Autodesk Inventor part; units mm, degrees
ref_plane "YZ Plane" through (0, 0, 0) normal (1, 0, 0) x (0, 1, 0)
ref_plane "XZ Plane" through (0, 0, 0) normal (0, 1, 0) x (-1, 0, 0)
ref_plane "XY Plane" through (0, 0, 0) normal (0, 0, 1) x (1, 0, 0)
sketch "スケッチ1" plane through (0, 0, 0) normal (0, 0, 1) x (1, 0, 0)
  line L0 (-22.5, 3.5) -> (22.5, 3.5)
  line L1 (22.5, 3.5) -> (22.5, -3.5)
  line L2 (22.5, -3.5) -> (-22.5, -3.5)
  line L3 (-22.5, -3.5) -> (-22.5, 3.5)
  line L4 (-22.5, 3.5) -> (22.5, -3.5) construction
  line L5 (22.5, 3.5) -> (-22.5, -3.5) construction
  line L6 (0, -6.37) -> (0, 6.37) construction
  line L7 (-34.37, 0) -> (34.37, 0) construction
  circle A0 centre (-20, 0) radius 4.55
  line L8 (22.5, -3.5) -> (22.5, 3.5)
  circle A1 centre (20, 0) radius 4.55
  circle A2 centre (-20, 0) radius 1.635
  circle A3 centre (20, 0) radius 1.635
  line L9 (14.5, 3.5) -> (14.5, -3.5)
  point P0 (0, 0)
  point P1 (-17.0927, 3.5)
  point P2 (-22.9073, 3.5)
  point P3 (-22.9073, -3.5)
  point P4 (-17.0927, -3.5)
  point P5 (17.0927, 3.5)
  point P6 (17.0927, -3.5)
  point P7 (22.9073, -3.5)
  point P8 (22.9073, 3.5)
  dimension "d1" = 7
  dimension "d2" = 20
  dimension "d3" = 45
  dimension "d4" = 9.1
  dimension "d12" = 3.27
  dimension "d13" = 8
  dimension "d16" = 3.27
extrude "押し出し1" add sketch "スケッチ1" along normal mid plane 5 contours L0 A0 L2 L3 | L0 L9 L2 A0 | L0 A1 L2 L9 | L0 L1 L2 A1 picked at (-19.7985, 2.8744) picked at (19.7985, -2.8744)
fillet "フィレット1" radius 3 4 edges at (-22.5, 3.5, 0) (-22.5, -3.5, 0) (22.5, -3.5, 0) (22.5, 3.5, 0)
extrude "押し出し3" cut sketch "スケッチ1" against normal blind 3 from surface at 2.5 contours L0 A1 L2 L9 | L0 L1 L2 A1 picked at (19.7985, -2.8744)
properties part number "link_arm_1"
Input: part model. Units: mm. Frame: model coordinates. A direction names the side the tool comes from. Give positions to 0.01 mm unless a question says otherwise; leave off trailing zeros. Write each loop counter-clockwise with the first axis right and the second up, starting at its lowest first coordinate (ties: lowest second). Pieces come first, ordered by that corner, then holes. Notation, with made-up numbers: (87, 77.25) -> (105, 77.25) arc R19 ccw to (105, 87.25) -> close; hole circle Ø4 at (-23, 15.5). An arc over 180 degrees is marked (long way). Use one line per item in the form item = value. Start each with the question number.
1) Section query D-D on x = -20. Return the cut outline in (y, z) (3 decimals), then the cut area to 3 significant figures.
2) Draft query along X for faces 3 (the cylindrical face through (21.51, 0.63, -1.51)), 4 (the flat face through (-4, 0, 2.5)), 5 (the flat face through (22.5, 0, -2)). Return one class per face: pulls with the +X half, pulls with the -X half, needs draft (parallel to the pull), parting line crosses it, or undercut.
3) Pin query (flat end, axial travel): pin 1 (2.5 mm diameter, centred on x = -20, y = 0, fed in from +Z); pin 2 (1 mm diameter, centred on y = -0.5, z = 2, fed in from +X). Return the tip coordinate at first contact, or that it passes through.
4) Section query C-C on z = 0.45. Return the cut outline in (x, y) (3 decimals), then the cut area to 3 significant figures.
5) Set-up query: faces 1 (the cylindrical face through (-21.6, 2.64, 0.04)), 2 (the flat face through (18, 0, -0.5)). Return all of +Z, -Z, +X, -X, +Y, -Y with unobstructed straight access to the full face (end or side cutting, diameter ignored); none if empty.
6) Section query A-A on y = 0. Return the cut outline in (x, z) (3 decimals), then the cut area to 3 significant figures.
7) Section query B-B on x = 20. Return the cut outline in (y, z) (3 decimals), then the cut area to 3 significant figures.
8) Ray query, probe 1 along Z at (x, y) = (20.5, -2.5); probe 2 along Y at (x, z) = (-20, 0.7) (3 decimals); probe 3 along X at (y, z) = (-0.25, -0.95). Return the intervals inside material, ascending. Write a range as from..to.
Outcome:
q1.outline = (-3.458, -2.5) -> (-1.635, -2.5) -> (-1.635, 2.5) -> (-3.458, 2.5) -> close; (1.635, -2.5) -> (3.458, -2.5) -> (3.458, 2.5) -> (1.635, 2.5) -> close
q1.area = 18.2 mm^2
q2.face_3 = undercut
q2.face_4 = needs draft
q2.face_5 = pulls with the +X half
q3.pin_1 = through
q3.pin_2 = 14.5
q4.outline = (-22.5, -0.5) arc R3 ccw to (-19.5, -3.5) -> (14.5, -3.5) -> (14.5, 3.5) -> (-19.5, 3.5) arc R3 ccw to (-22.5, 0.5) -> close; hole circle Ø3.27 at (-20, 0)
q4.area = 247 mm^2
q5.face_1 = +Z, -Z, -X, +Y
q5.face_2 = +Z, +X, +Y, -Y
q6.outline = (-22.5, -2.5) -> (-21.635, -2.5) -> (-21.635, 2.5) -> (-22.5, 2.5) -> close; (-18.365, -2.5) -> (18.365, -2.5) -> (18.365, -0.5) -> (14.5, -0.5) -> (14.5, 2.5) -> (-18.365, 2.5) -> close; (21.635, -2.5) -> (22.5, -2.5) -> (22.5, -0.5) -> (21.635, -0.5) -> close
q6.area = 178 mm^2
q7.outline = (-3.458, -2.5) -> (-1.635, -2.5) -> (-1.635, -0.5) -> (-3.458, -0.5) -> close; (1.635, -2.5) -> (3.458, -2.5) -> (3.458, -0.5) -> (1.635, -0.5) -> close
q7.area = 7.29 mm^2
q8.probe_1 = -2.5..-0.5
q8.probe_2 = -3.458..-1.635, 1.635..3.458
q8.probe_3 = -22.5..-21.62, -18.38..18.38, 21.62..22.5
